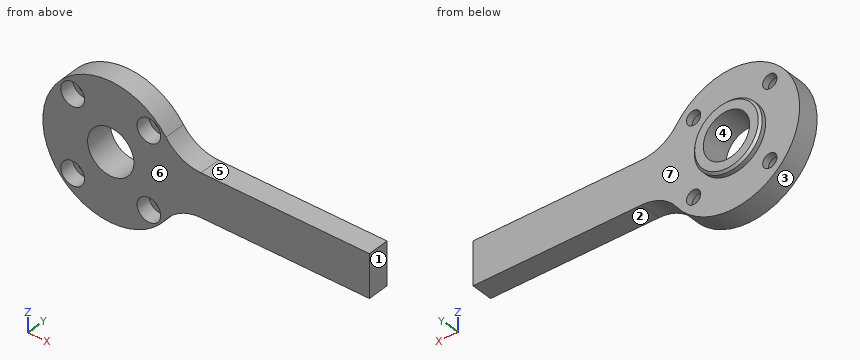
```python
from build123d import *

# Parameters (mm, degrees)
SKETCH_2_R          = 31.5
EXTRUDE_1_DEPTH     = 10
SKETCH_3_R          = 15.75
EXTRUDE_2_DEPTH     = 3
SKETCH_5_R          = 3.3
CUT_EXTRUDE_2_DEPTH = 47.405818601
SKETCH_5_3_R        = 5.5
CUT_EXTRUDE_3_DEPTH = 6.8
SKETCH_6_W          = 20
SKETCH_6_H          = 10
EXTRUDE_3_DEPTH     = 120
SKETCH_4_R          = 10.75
CUT_EXTRUDE_4_DEPTH = 125.744739368
CHAMFER_1_SIZE      = 1
FILLET_1_R          = 20
FILLET_2_R          = 20


with BuildPart() as part:
    # Sketch 2 → Extrude 1 (new body)
    with BuildSketch(Plane(origin=(0, 0, 0), x_dir=(1, 0, 0), z_dir=(0, 1, 0))):
        with Locations(Location((0, 0, 0), (0, 0, 270))):
            Circle(SKETCH_2_R)
    extrude(amount=EXTRUDE_1_DEPTH)

    # Sketch 3 → Extrude 2 (add)
    with BuildSketch(Plane(origin=(0, 10, 0), x_dir=(1, 0, 0), z_dir=(0, 1, 0))):
        with Locations(Location((0, 0, 0), (0, 0, 270))):
            Circle(SKETCH_3_R)
    extrude(amount=EXTRUDE_2_DEPTH)

    # Sketch 5 → Cut-Extrude 2 (cut, through all)
    with BuildSketch(Plane.XZ):
        with Locations(Location((17.67766953, 17.67766953, 0), (0, 0, 270))):
            Circle(SKETCH_5_R)
        with Locations(Location((-17.67766953, 17.67766953, 0), (0, 0, 90))):
            Circle(SKETCH_5_R)
        with Locations(Location((-17.67766953, -17.67766953, 0), (0, 0, 270))):
            Circle(SKETCH_5_R)
        with Locations(Location((17.67766953, -17.67766953, 0), (0, 0, 90))):
            Circle(SKETCH_5_R)
    extrude(amount=-CUT_EXTRUDE_2_DEPTH, mode=Mode.SUBTRACT)

    # Sketch 5_3 → Cut-Extrude 3 (cut)
    with BuildSketch(Plane.XZ):
        with Locations(Location((17.67766953, 17.67766953, 0), (0, 0, 270))):
            Circle(SKETCH_5_3_R)
        with Locations(Location((-17.67766953, 17.67766953, 0), (0, 0, 90))):
            Circle(SKETCH_5_3_R)
        with Locations(Location((-17.67766953, -17.67766953, 0), (0, 0, 270))):
            Circle(SKETCH_5_3_R)
        with Locations(Location((17.67766953, -17.67766953, 0), (0, 0, 90))):
            Circle(SKETCH_5_3_R)
    extrude(amount=-CUT_EXTRUDE_3_DEPTH, mode=Mode.SUBTRACT)

    # Sketch 6 → Extrude 3 (add)
    with BuildSketch(Plane(origin=(0, 0, 0), x_dir=(0, 0, -1), z_dir=(1, 0, 0))):
        with Locations((0, 5)):
            Rectangle(SKETCH_6_W, SKETCH_6_H)
    extrude(amount=EXTRUDE_3_DEPTH)

    # Sketch 4 → Cut-Extrude 4 (cut, through all)
    with BuildSketch(Plane(origin=(0, 0, 0), x_dir=(-1, 0, 0), z_dir=(0, -1, 0))):
        with Locations(Location((0, 0, 0), (0, 0, 90))):
            Circle(SKETCH_4_R)
    extrude(amount=-CUT_EXTRUDE_4_DEPTH, mode=Mode.SUBTRACT)

    # Chamfer 1
    chamfer_1_edges = [part.edges().sort_by_distance(p)[0] for p in [
        (0, 13, -15.75),
    ]]
    chamfer(chamfer_1_edges, length=CHAMFER_1_SIZE)

    # Fillet 1
    fillet_1_edges = [part.edges().sort_by_distance(p)[0] for p in [
        (29.870554062, 5, -10),
    ]]
    fillet(fillet_1_edges, radius=FILLET_1_R)

    # Fillet 2
    fillet_2_edges = [part.edges().sort_by_distance(p)[0] for p in [
        (29.870554062, 5, 10),
    ]]
    fillet(fillet_2_edges, radius=FILLET_2_R)


solid = part.part
```
Geometry check sheet. Reference: the model listing, model coordinates, mm. Face numbers are marked on the shaded views. A direction names the side the tool comes from. Give positions to 0.01 mm unless a question says otherwise; leave off trailing zeros. Loops run counter-clockwise (first coordinate to the right, second up) from the corner with the lowest first, then second, coordinate; pieces in that order, holes last. Notation, with made-up numbers: M -26,30 L 20,30 A17 cw 20,52 Z; hole C 11,25 d5. An arc over 180 degrees is marked long. Write item = value, one per line. Start each with the question number.
1. Draft check along X on the marked faces 1, 2, 3 and 4. Enter one of: +X half, -X half, draft (parallel to the pull), parting line (faces both ways), or undercut.
2. Section check A-A, the plane x = 0. Enter the section's corners in (y, z), plus the area to 3 significant figures.
3. Thickness scan on probe 1 along X at (y, z) = (1, 18); probe 2 along X at (y, z) = (2.5, 19.5); probe 3 along Y at (x, z) = (55.5, -4.5). Record the ranges inside material, lowest first.
4. Section check D-D, the plane x = 93.5. Enter the section's corners in (y, z), plus the area to 3 significant figures.
5. Go/stop test with flat-tipped pins: P1, Ø12.5, axis at x = 17.68, z = 17.68, coming from the +Y side; P2, Ø2, axis at x = -15, y = 6.5, coming from the +Z side; P3, Ø3, axis at x = 80.5, y = 5, coming from the -Z side; P4, Ø5.5, axis at x = -17.68, z = 17.68, coming from the +Y side. Record where each tip stops, or that it passes through.
6. Section check C-C, the plane y = 4. Enter the section's corners in (x, z).
7. Tool access check on the marked faces 5, 6 and 7. Record the directions out of +Z, -Z, +X, -X, +Y, -Y that give a thin tool (end or side, any length) a straight path to the whole face; none if there is none.
8. Section check B-B, the plane z = 0. Enter the section's corners in (x, y), plus the area to 3 significant figures.
Values follow:
q1.face_1 = +X half
q1.face_2 = draft
q1.face_3 = parting line
q1.face_4 = undercut
q2.outline = M 0,-31.5 L 10,-31.5 L 10,-15.75 L 12,-15.75 L 13,-14.75 L 13,-10.75 L 0,-10.75 Z; M 0,10.75 L 13,10.75 L 13,14.75 L 12,15.75 L 10,15.75 L 10,31.5 L 0,31.5 Z
q2.area = 444 mm^2
q3.probe_1 = -25.85 to -23.17, -12.19 to 12.19, 23.17 to 25.86
q3.probe_2 = -24.74 to -22.87, -12.49 to 12.49, 22.87 to 24.74
q3.probe_3 = 0 to 10
q4.outline = M 0,-10 L 10,-10 L 10,10 L 0,10 Z
q4.area = 200 mm^2
q5.P1 = 10
q5.P2 = 28.22
q5.P3 = -10
q5.P4 = through
q6.outline = M 25.6,-18.35 A20 cw 41.86,-10 L 120,-10 L 120,10 L 41.86,10 A20 cw 25.6,18.35 A31.5 ccw long Z; hole C -17.68,-17.68 d11; hole C -17.68,17.68 d11; hole C 0,0 d21.5; hole C 17.68,-17.68 d11; hole C 17.68,17.68 d11
q7.face_5 = +Z, +X, +Y, -Y
q7.face_6 = +Z, -Z, +X, -X, -Y
q7.face_7 = +Y
q8.outline = M -31.5,0 L -10.75,0 L -10.75,13 L -14.75,13 L -15.75,12 L -15.75,10 L -31.5,10 Z; M 10.75,0 L 120,0 L 120,10 L 15.75,10 L 15.75,12 L 14.75,13 L 10.75,13 Z
q8.area = 1,330 mm^2
